Autodesk Inventor part; units mm, degrees
ref_plane "YZ Plane" through (0, 0, 0) normal (1, 0, 0) x (0, 1, 0)
ref_plane "XZ Plane" through (0, 0, 0) normal (0, 1, 0) x (-1, 0, 0)
ref_plane "XY Plane" through (0, 0, 0) normal (0, 0, 1) x (1, 0, 0)
sketch "スケッチ1" plane through (0, 0, 0) normal (0, 1, 0) x (-1, 0, 0)
  circle A0 centre (0, 5) radius 1.6
  circle A1 centre (0, -5) radius 1.6
  line L0 (5.6, 0) -> (-5.6, 0)
  line L1 (0, -5) -> (0, 5) construction
  line L2 (4, -5) -> (4, 5)
  line L3 (-4, 5) -> (-4, -5)
  arc A2 (-4, -5) -> (4, -5) centre (0, -5) ccw
  arc A3 (4, 5) -> (-4, 5) centre (0, 5) ccw
  point P0 (0, 0)
  dimension "d0" = 3.2
  dimension "d1" = 3.2
  dimension "d2" = 10
  dimension "d3" = 4
extrude "押し出し1" add sketch "スケッチ1" along normal blind 10.5
properties part number "spacer_2_hole"
Could you check a few things on this model? Use its own coordinates, in mm. Coordinates: 2 decimals unless noted, no trailing zeros. Write each loop counter-clockwise with the first axis right and the second up, starting at its lowest first coordinate (ties: lowest second). Pieces come first, ordered by that corner, then holes. Notation, with made-up numbers: M -24.5,35.25 L 11.5,35.25 A24 cw 11.5,62.25 Z; hole C 66,0.25 d2. An arc over 180 degrees is marked long. Answer as CSV lines item,"result". Start each with the question number.
1) I want a section at C-C, the plane x = 3. Please give me the cut outline in (y, z).
2) I want a section at B-B, the plane y = 6.25. Please give me the cut outline in (x, z).
3) I want a section at D-D, the plane z = -7. Please give me the cut outline in (x, y), and give its area (3 significant figures).
4) I want a section at A-A, the plane x = 0. Please give me the cut outline in (y, z), and give its area (3 significant figures).
5) Please list where these lines run through material, in increasing order: line 1 (Z direction, x = 0, y = 4.25); line 2 (Z direction, x = 1, y = 8.5); line 3 (X direction, y = 4.75, z = -5.5). Write a range as from..to.
6) We'd pull the mould along Z, two halves only. Please class faces 1 (the flat face through (0, 0, 0)), 2 (the cylindrical face through (0, 5, 9)), 3 (the cylindrical face through (0.35, 5.18, 6.56)): +Z half, -Z half, draft (parallel to the pull), parting line (faces both ways), or undercut.
7) For P1, Ø4, axis at x = 1.5, z = -5, coming from the +Y side; P2, Ø2.5, axis at x = 0, z = 5, coming from the +Y side, each with a flat end and sliding along its axis, tell me the tip position at first contact or that it passes through.
Data:
1,outline,"M 0,-7.65 L 10.5,-7.65 L 10.5,7.65 L 0,7.65 Z"
2,outline,"M -4,-5 A4 ccw 4,-5 L 4,5 A4 ccw -4,5 Z; hole C 0,-5 d3.2; hole C 0,5 d3.2"
3,outline,"M -3.46,0 L 3.46,0 L 3.46,10.5 L -3.46,10.5 Z"
3,area,"72.7 mm^2"
4,outline,"M 0,-9 L 10.5,-9 L 10.5,-6.6 L 0,-6.6 Z; M 0,-3.4 L 10.5,-3.4 L 10.5,3.4 L 0,3.4 Z; M 0,6.6 L 10.5,6.6 L 10.5,9 L 0,9 Z"
4,area,"122 mm^2"
5,line 1,"z = -9..-6.6, -3.4..3.4, 6.6..9"
5,line 2,"z = -8.87..-6.25, -3.75..3.75, 6.25..8.87"
5,line 3,"x = -3.97..-1.52, 1.52..3.97"
6,face 1,"draft"
6,face 2,"+Z half"
6,face 3,"undercut"
7,P1,"stops at y = 10.5"
7,P2,"passes through"
